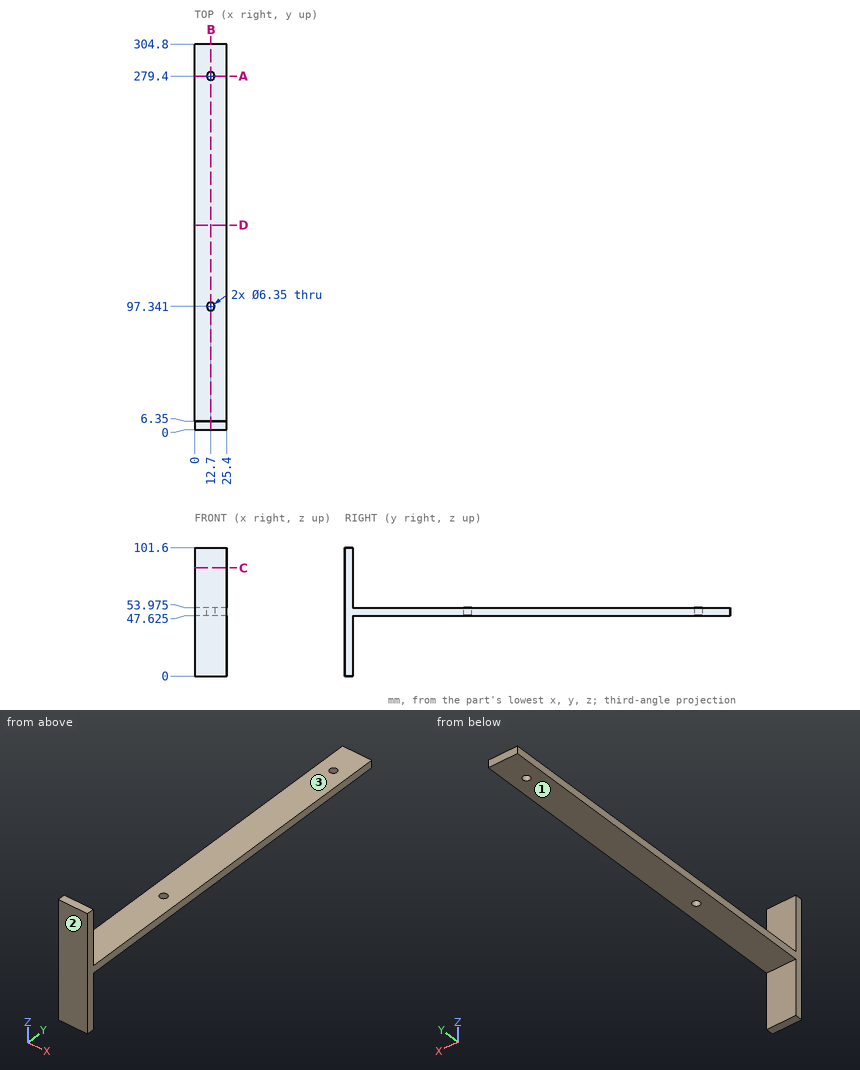
For this review, use the dimensioned drawing (mm, ordinates from the lowest corner) and the shaded views. A direction names the side the tool comes from. Round coordinates to 2 decimals unless told otherwise and drop trailing zeros. Write each loop counter-clockwise with the first axis right and the second up, starting at its lowest first coordinate (ties: lowest second). Pieces come first, ordered by that corner, then holes. Notation, with made-up numbers: (57.25, 51.5) -> (89.25, 51.5) arc R23 ccw to (89.25, 69.5) -> close; hole circle Ø3 at (-29.75, 34.25). An arc over 180 degrees is marked (long way). One line per item, written item: value. Start each with the question number.
Q1. Add section B-B (x = 12.7). State how many separate pieces and enclosed holes the cut face has, then the cut area to 3 significant figures.
Q2. To check wall thickness, follow probe 1 along Y at (x, z) = (12.7, 51) (1 decimal); probe 2 along Z at (x, y) = (11.25, 276.5) (1 decimal); probe 3 along Y at (x, z) = (10.25, 82). State the ranges of each line that lie inside material, in increasing order.
Q3. Insertion check: P1, Ø12.5, axis at x = 9, y = 217, coming from the +Z side (3 decimals); P2, Ø10, axis at x = 12.7, y = 97.34, coming from the -Z side (3 decimals); P3, Ø12.5, axis at x = 6.5, z = 14, coming from the +Y side. Each pin has a flat end and moves straight along its axis. Give the tip position at first contact, or say it passes through.
Q4. Add section D-D (y = 161.5). Give the boundary of the cut face in (x, z) (1 decimal).
Q5. Add section C-C (z = 85.5). Give the boundary of the cut face in (x, y).
Q6. Tool access review of the marked faces 1, 2 and 3: name each direction out of +Z, -Z, +X, -X, +Y, -Y from which nothing blocks a thin tool from reaching the whole face with its end or side.
Q7. Add section A-A (y = 279.4). Give the boundary of the cut face in (x, z) (1 decimal).
Response:
1. separate pieces: 3
1. enclosed holes: 0
1. area: 2,460 mm^2
2. probe 1: y = 0 to 94.2, 100.5 to 276.2, 282.6 to 304.8
2. probe 2: z = 47.6 to 54
2. probe 3: y = 0 to 6.35
3. P1: stops at z = 53.975
3. P2: stops at z = 47.625
3. P3: stops at y = 6.35
4. outline: (0, 47.6) -> (25.4, 47.6) -> (25.4, 54) -> (0, 54) -> close
5. outline: (0, 0) -> (25.4, 0) -> (25.4, 6.35) -> (0, 6.35) -> close
6. face 1: -Z, +X, -X, +Y
6. face 2: +Z, -Z, +X, -X, -Y
6. face 3: +Z, +X, -X, +Y
7. outline: (0, 47.6) -> (9.5, 47.6) -> (9.5, 54) -> (0, 54) -> close; (15.9, 47.6) -> (25.4, 47.6) -> (25.4, 54) -> (15.9, 54) -> close
